```python
from build123d import *

# Parameters (mm, degrees)
SALIENTE_EXTRUIR1_DEPTH = 3


with BuildPart() as part:
    # Croquis1 → Saliente-Extruir1 (new body)
    with BuildSketch(Plane(origin=(0, 0, 0), x_dir=(1, 0, 0), z_dir=(0, 1, 0))):
        Polygon((12.5, 3), (12.5, 0), (22.5, 0), (22.5, 3), (32.5, 3), (32.5, 0), (42.5, 0), (42.5, 3), (52.5, 3), (52.5, 0), (62.5, 0), (62.5, 3), (72, 3), (72, 5), (75, 5), (75, 8), (72, 8), (72, 10), (62.5, 10), (62.5, 13), (52.5, 13), (52.5, 10), (42.5, 10), (42.5, 13), (37.5, 13), (32.5, 13), (32.5, 10), (22.5, 10), (22.5, 13), (12.5, 13), (12.5, 10), (3, 10), (3, 8), (0, 8), (0, 6.5), (0, 5), (3, 5), (3, 3), align=None)
    extrude(amount=SALIENTE_EXTRUIR1_DEPTH)


solid = part.part
```
Design review of the part built by this model. Coordinates are the model's own, in mm. A direction names the side the tool comes from. Coordinates: 2 decimals unless noted, no trailing zeros. Order: outer loops, then holes, each group sorted by start corner. A loop starts at its lowest first (then second) coordinate and runs counter-clockwise, first axis right, second up. Notation, with made-up numbers: M 37.5,55.5 L 68.5,55.5 A27 ccw 68.5,86.5 Z; hole C -20.5,68 d1. An arc over 180 degrees is marked long. Answer as a JSON object with one key per item and string values. Group by question number.
1) For pin 1 (0.9 mm diameter, centred on x = 1, y = 1, fed in from +Z); pin 2 (1.5 mm diameter, centred on y = 2, z = -11, fed in from -X); pin 3 (0.9 mm diameter, centred on x = 73.5, y = 1, fed in from -Z), all flat-tipped, find the tip position at first contact; note any pin that passes through.
2) Wall thickness on L1, parallel to X at y = 0.3, z = -12; L2, parallel to X at y = 2.8, z = -3.5; L3, parallel to Z at x = 4, y = 0.3: over which ranges is each line inside the solid? List them lowest first.
3) Mouldability with a two-part tool opening along X and no side actions: class faces 1 (the flat face through (22.5, 1, -1)), 2 (the flat face through (74, 1, -8)), 3 (the flat face through (0, 1, -7)) as pulls with the +X half, pulls with the -X half, needs draft (parallel to the pull), parting line crosses it, or undercut.
4) Add section A-A, the plane z = -1.5. Write out the cut boundary in (x, y).
5) Add section B-B, the plane z = -4.25. Write out the cut boundary in (x, y), then the cut area to 3 significant figures.
6) Tool access review of faces 4 (the flat face through (12.5, 1, -2)), 5 (the flat face through (12.5, 1, -12)), 6 (the flat face through (32.5, 1, -12)), 7 (the flat face through (72, 1, -9)): name each direction out of +Z, -Z, +X, -X, +Y, -Y from which nothing blocks a thin tool from reaching the whole face with its end or side.
7) Add section C-C, the plane x = 69.5. Write out the cut boundary in (y, z), then the cut area to 3 significant figures.
Computed values:
{
 "1": {"pin 1": "stops at z = -5", "pin 2": "stops at x = 12.5", "pin 3": "stops at z = -8"},
 "2": {"L1": "x = 12.5 to 22.5, 32.5 to 42.5, 52.5 to 62.5", "L2": "x = 3 to 72", "L3": "z = -10 to -3"},
 "3": {"face 1": "undercut", "face 2": "needs draft", "face 3": "pulls with the -X half"},
 "4": {"outline": "M 12.5,0 L 22.5,0 L 22.5,3 L 12.5,3 Z; M 32.5,0 L 42.5,0 L 42.5,3 L 32.5,3 Z; M 52.5,0 L 62.5,0 L 62.5,3 L 52.5,3 Z"},
 "5": {"outline": "M 3,0 L 72,0 L 72,3 L 3,3 Z", "area": "207 mm^2"},
 "6": {"face 4": "+Z, -X, +Y, -Y", "face 5": "-Z, -X, +Y, -Y", "face 6": "-Z, +Y, -Y", "face 7": "-Z, +X, +Y, -Y"},
 "7": {"outline": "M 0,-10 L 3,-10 L 3,-3 L 0,-3 Z", "area": "21.0 mm^2"}
}
